The model under review builds one solid part; all positions refer to its coordinate system, in mm. A direction names the side the tool comes from. Coordinates: 2 decimals unless noted, no trailing zeros. Loops run counter-clockwise (first coordinate to the right, second up) from the corner with the lowest first, then second, coordinate; pieces in that order, holes last. Notation, with made-up numbers: M 23,10 L 46,10 A20 cw 46,35 Z; hole C 25,50 d9. An arc over 180 degrees is marked long. Use one line per item in the form item = value.
```python
from build123d import *

# Parameters (mm, degrees)
SKETCH_1_W     = 23
SKETCH_1_H     = 8.25
SKETCH_2_R     = 10
F_02_HEX_DEPTH = 6


with BuildPart() as part:
    # 草图1 → 01_SLEEVE (revolve)
    with BuildSketch(Plane.XY, mode=Mode.PRIVATE) as f_01_sleeve_sk:
        with Locations((11.5, 14.125)):
            Rectangle(SKETCH_1_W, SKETCH_1_H)
    revolve(f_01_sleeve_sk.sketch.rotate(Axis((-5, 0, 0), (1, 0, 0)), 90), axis=Axis((-5, 0, 0), (1, 0, 0)))

    # 草图2 → 02_HEX (add)
    with BuildSketch(Plane(origin=(23, 0, 0), x_dir=(0, 0, -1), z_dir=(1, 0, 0))):
        Polygon((18.475208614, 0), (9.237604307, 16), (-9.237604307, 16), (-18.475208614, 0), (-9.237604307, -16), (9.237604307, -16), align=None)
        with Locations(Location((0, 0, 0), (0, 0, 180))):
            Circle(SKETCH_2_R, mode=Mode.SUBTRACT)
    extrude(amount=F_02_HEX_DEPTH)


solid = part.part
```
1. Wall thickness on line 1 along Y through (x, z) = (15.25, 0); line 2 along Z through (x, y) = (14.25, -1.5); line 3 along X through (y, z) = (11.5, 12): over which ranges is each line inside the solid? List them lowest first. Write a range as from..to.
Response values:
line_1 = -18.25..-10, 10..18.25
line_2 = -18.19..-9.89, 9.89..18.19
line_3 = 0..23
2. Add section B-B (x = 24.25). State the section outline as (y, z) points.
Response values:
outline = M -16,-9.24 L 0,-18.48 L 16,-9.24 L 16,9.24 L 0,18.48 L -16,9.24 Z; hole C 0,0 d20
3. Add section D-D (y = -15). State the section outline as (x, z) points, then the cut area to 3 significant figures.
Response values:
outline = M 0,-10.4 L 23,-10.4 L 23,-9.81 L 29,-9.81 L 29,9.81 L 23,9.81 L 23,10.4 L 0,10.4 Z
area = 596 mm^2
4. Add section A-A (z = 0). State the section outline as (x, y) points, then the cut area to 4 significant figures.
Response values:
outline = M 0,-18.25 L 23,-18.25 L 23,-16 L 29,-16 L 29,-10 L 0,-10 Z; M 0,10 L 29,10 L 29,16 L 23,16 L 23,18.25 L 0,18.25 Z
area = 451.5 mm^2
5. The part is to be moulded in two halves that separate along Y. For faces 5 (the face through (14, 0, -10)), 6 (the face through (23, -9, -15)), 7 (the face through (26, 8.1, 13.8)), say which applies: pulls with the +Y half, pulls with the -Y half, needs draft (parallel to the pull), parting line crosses it, or undercut.
Response values:
face_5 = undercut
face_6 = needs draft
face_7 = pulls with the +Y half
6. Machinability: for faces 1 (the face through (23, 9, 15)), 2 (the face through (26, -8.1, -13.8)), 3 (the face through (25.96, -7.89, 13.92)), 4 (the face through (26, 16, 0)), which of the approach directions +Z, -Z, +X, -X, +Y, -Y give a long, thin tool a straight path to every point of the face, cutting with its end or side? Answer none if there is none.
Response values:
face_1 = +Z, +X, +Y
face_2 = -Z, +X, -Y
face_3 = +Z, +X, -Y
face_4 = +Z, -Z, +X, +Y
7. Insertion check: P1, Ø1, axis at x = 24.5, z = -11, coming from the +Y side; P2, Ø1.1, axis at y = -16.5, z = -1, coming from the +X side; P3, Ø10, axis at x = 12.5, y = 13, coming from the +Z side; P4, Ø1, axis at x = 3.5, y = 13.5, coming from the -Z side. Each pin has a flat end and moves straight along its axis. Give the tip position at first contact, or say it passes through.
Response values:
P1 = 13.81
P2 = 29
P3 = 16.4
P4 = -12.81
8. Add section C-C (y = 8.5). State the section outline as (x, z) points.
Response values:
outline = M 0,-16.15 L 23,-16.15 L 23,-13.57 L 29,-13.57 L 29,-5.27 L 0,-5.27 Z; M 0,5.27 L 29,5.27 L 29,13.57 L 23,13.57 L 23,16.15 L 0,16.15 Z
